from build123d import *

# Parameters (mm, degrees)
ESQUISSE1_R        = 11.975
ESQUISSE1_R_2      = 9.5
BOSS_EXTRU_1_DEPTH = 2
ESQUISSE3_R        = 15
ESQUISSE3_W        = 15.5
ESQUISSE3_H        = 18
BOSS_EXTRU_5_DEPTH = 2
ESQUISSE8_R        = 15
ESQUISSE8_W        = 15.5
ESQUISSE8_H        = 18
BOSS_EXTRU_6_DEPTH = 4


with BuildPart() as part:
    # Esquisse1 → Boss.-Extru.1 (new body)
    with BuildSketch(Plane(origin=(0, 0, 0), x_dir=(1, 0, 0), z_dir=(0, 1, 0))):
        Circle(ESQUISSE1_R)
        Circle(ESQUISSE1_R_2, mode=Mode.SUBTRACT)
    extrude(amount=BOSS_EXTRU_1_DEPTH)

    # Esquisse3 → Boss.-Extru.5 (add)
    with BuildSketch(Plane(origin=(0, 2, 0), x_dir=(1, 0, 0), z_dir=(0, 1, 0))):
        Circle(ESQUISSE3_R)
        Rectangle(ESQUISSE3_W, ESQUISSE3_H, mode=Mode.SUBTRACT)
    extrude(amount=BOSS_EXTRU_5_DEPTH)

    # Esquisse8 → Boss.-Extru.6 (add)
    with BuildSketch(Plane(origin=(0, 4, 0), x_dir=(1, 0, 0), z_dir=(0, 1, 0))):
        Circle(ESQUISSE8_R)
        Rectangle(ESQUISSE8_W, ESQUISSE8_H, mode=Mode.SUBTRACT)
    extrude(amount=BOSS_EXTRU_6_DEPTH)


solid = part.part
The listing builds one solid part. Answer for the finished solid, in the listing's coordinates (mm). A direction names the side the tool comes from. Coordinates: 2 decimals unless noted, no trailing zeros. Loops run counter-clockwise (first coordinate to the right, second up) from the corner with the lowest first, then second, coordinate; pieces in that order, holes last. Notation, with made-up numbers: (-22, -18) -> (11, -18) arc R24 cw to (11, -4) -> close; hole circle Ø9 at (-27.5, 29.25). An arc over 180 degrees is marked (long way). Answer in a Markdown table with one row per item. Add a question column.
1. For faces 1 (the flat face through (0, 5, 9)), 2 (the flat face through (8, 2, 0)), 3 (the flat face through (-4, 0, -9)), determine the directions among +Z, -Z, +X, -X, +Y, -Y from which every point of the face is accessible in a straight line to the end or side of a thin tool.
2. Consider line 1 (X direction, y = 1.1, z = 0) (3 decimals); line 2 (X direction, y = 3.25, z = 2.75). Determine where each line is inside the solid, lowest interval first. Write a range as [from, to].
3. Flat-ended cylindrical pins translate along their axes: P1, Ø4, axis at x = 5, z = 6.5, coming from the +Y side; P2, Ø3, axis at y = 6.5, z = -2.5, coming from the -X side; P3, Ø1, axis at x = 9, y = 6.5, coming from the -Z side; P4, Ø12, axis at x = 9.5, z = -0.5, coming from the -Y side. Find the tip coordinate at first contact, or state that the pin passes through.
4. The part is cut by section C-C, the plane y = 4.75. Write down the section's boundary in (x, z), then the cut area to 3 significant figures.
5. The part is cut by section A-A, the plane x = 0. Write down the section's boundary in (y, z) (3 decimals).
6. Determine the mould class of faces 4 (the flat face through (0, 5, -9)), 5 (the flat face through (-8, 2, 0)), 6 (the cylindrical face through (-14.985, 4.958, -0.66)), 7 (the flat face through (-10, 2, 7)) for opening direction X: +X half, -X half, draft (parallel to the pull), parting line (faces both ways), or undercut.
7. The part is cut by section B-B, the plane z = 0. Write down the section's boundary in (x, y) (3 decimals).
8. The part is cut by section D-D, the plane z = -10.75. Write down the section's boundary in (x, y).
Answer below:
| question | item | result |
|---|---|---|
| 1 | face 1 | +Y |
| 1 | face 2 | -Y |
| 1 | face 3 | +Z, -Z, +X, -X, -Y |
| 2 | line 1 | [-11.975, -9.5], [9.5, 11.975] |
| 2 | line 2 | [-14.75, -7.75], [7.75, 14.75] |
| 3 | P1 | y = 2 |
| 3 | P2 | x = -14.97 |
| 3 | P3 | z = -12.36 |
| 3 | P4 | y = 0 |
| 4 | outline | circle Ø30 at (0, 0); hole (-7.75, -9) -> (7.75, -9) -> (7.75, 9) -> (-7.75, 9) -> close |
| 4 | area | 428 mm2 |
| 5 | outline | (0, -11.975) -> (2, -11.975) -> (2, -15) -> (8, -15) -> (8, -9) -> (2, -9) -> (2, -9.5) -> (0, -9.5) -> close; (0, 9.5) -> (2, 9.5) -> (2, 9) -> (8, 9) -> (8, 15) -> (2, 15) -> (2, 11.975) -> (0, 11.975) -> close |
| 6 | face 4 | undercut |
| 6 | face 5 | undercut |
| 6 | face 6 | parting line |
| 6 | face 7 | draft |
| 7 | outline | (-15, 2) -> (-11.975, 2) -> (-11.975, 0) -> (-9.5, 0) -> (-9.5, 2) -> (-7.75, 2) -> (-7.75, 8) -> (-15, 8) -> close; (7.75, 2) -> (9.5, 2) -> (9.5, 0) -> (11.975, 0) -> (11.975, 2) -> (15, 2) -> (15, 8) -> (7.75, 8) -> close |
| 8 | outline | (-10.46, 2) -> (-5.28, 2) -> (-5.28, 0) -> (5.28, 0) -> (5.28, 2) -> (10.46, 2) -> (10.46, 8) -> (-10.46, 8) -> close |
